Design review of the part shown in the three views and the two pictorial views. Dimensions are in mm from the part's minimum x, y and z. Give positions to 0.01 mm unless a question says otherwise; leave off trailing zeros. Order: outer loops, then holes, each group sorted by start corner. A loop starts at its lowest first (then second) coordinate and runs counter-clockwise, first axis right, second up. Notation, with made-up numbers: (11.25, -32.75) -> (27.25, -32.75) arc R18 ccw to (27.25, -15.75) -> close; hole circle Ø5 at (4.5, -27). An arc over 180 degrees is marked (long way). Answer in a Markdown table with one row per item. Add a question column.
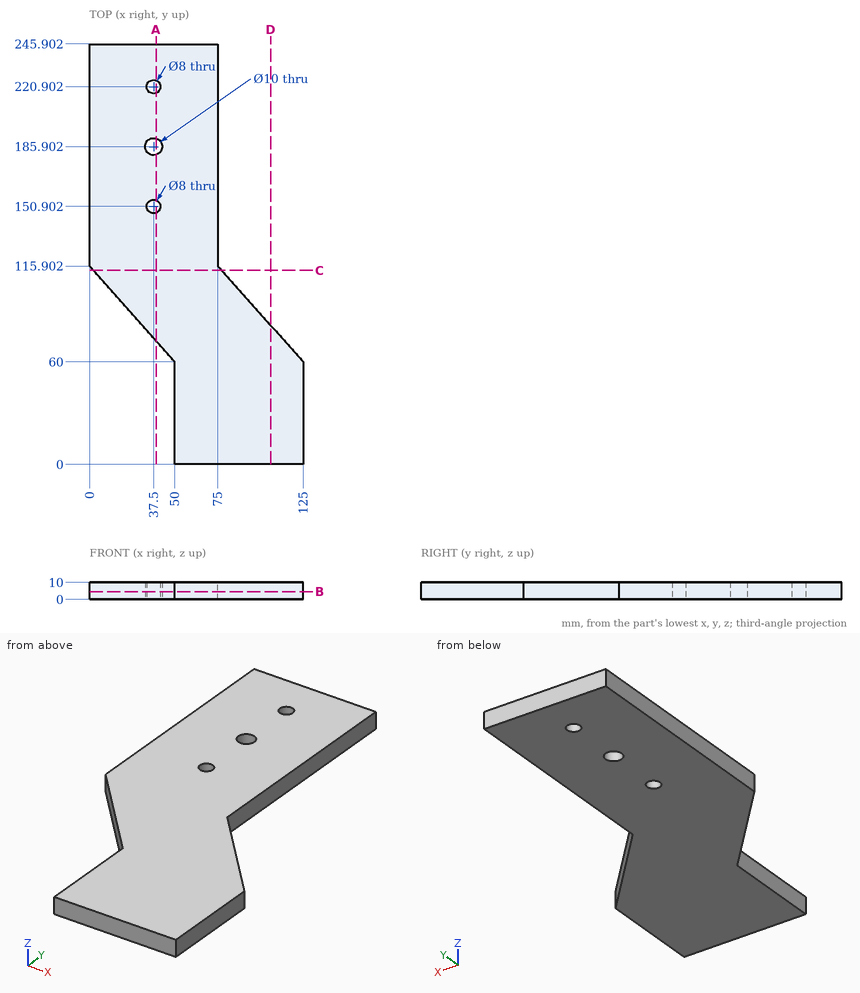
1) For L1, parallel to Y at x = 37.5, z = 6.5 (1 decimal); L2, parallel to X at y = 30, z = 2.5; L3, parallel to X at y = 182, z = 1.25 (1 decimal), list the stretches that pass through material, from the lowest coordinate up.
2) Clearance check with flat-ended pins moving along their axes: P1, Ø3, axis at y = 203, z = 3, coming from the +X side; P2, Ø9, axis at x = 37.5, y = 150.9, coming from the +Z side; P3, Ø2, axis at x = 104.5, z = 5, coming from the +Y side; P4, Ø3, axis at y = 30, z = 7, coming from the -X side. State where each tip first meets the part, or that it passes through.
3) Add section A-A, the plane x = 39. Write out the cut boundary in (y, z), and give its area (3 significant figures).
4) Add section B-B, the plane z = 4.5. Write out the cut boundary in (x, y), and give its area (3 significant figures).
5) Add section C-C, the plane y = 113.5. Write out the cut boundary in (x, z).
6) Add section D-D, the plane x = 106. Write out the cut boundary in (y, z).
Verdict:
| question | item | result |
|---|---|---|
| 1 | L1 | y = 74 to 146.9, 154.9 to 180.9, 190.9 to 216.9, 224.9 to 245.9 |
| 1 | L2 | x = 50 to 125 |
| 1 | L3 | x = 0 to 34.4, 40.6 to 75 |
| 2 | P1 | stops at x = 75 |
| 2 | P2 | stops at z = 10 |
| 2 | P3 | stops at y = 84.04 |
| 2 | P4 | stops at x = 50 |
| 3 | outline | (72.3, 0) -> (147.19, 0) -> (147.19, 10) -> (72.3, 10) -> close; (154.61, 0) -> (181.13, 0) -> (181.13, 10) -> (154.61, 10) -> close; (190.67, 0) -> (217.19, 0) -> (217.19, 10) -> (190.67, 10) -> close; (224.61, 0) -> (245.9, 0) -> (245.9, 10) -> (224.61, 10) -> close |
| 3 | area | 1,490 mm2 |
| 4 | outline | (0, 115.9) -> (50, 60) -> (50, 0) -> (125, 0) -> (125, 60) -> (75, 115.9) -> (75, 245.9) -> (0, 245.9) -> close; hole circle Ø10 at (37.5, 185.9); hole circle Ø8 at (37.5, 150.9); hole circle Ø8 at (37.5, 220.9) |
| 4 | area | 18,300 mm2 |
| 5 | outline | (2.15, 0) -> (77.15, 0) -> (77.15, 10) -> (2.15, 10) -> close |
| 6 | outline | (0, 0) -> (81.24, 0) -> (81.24, 10) -> (0, 10) -> close |
